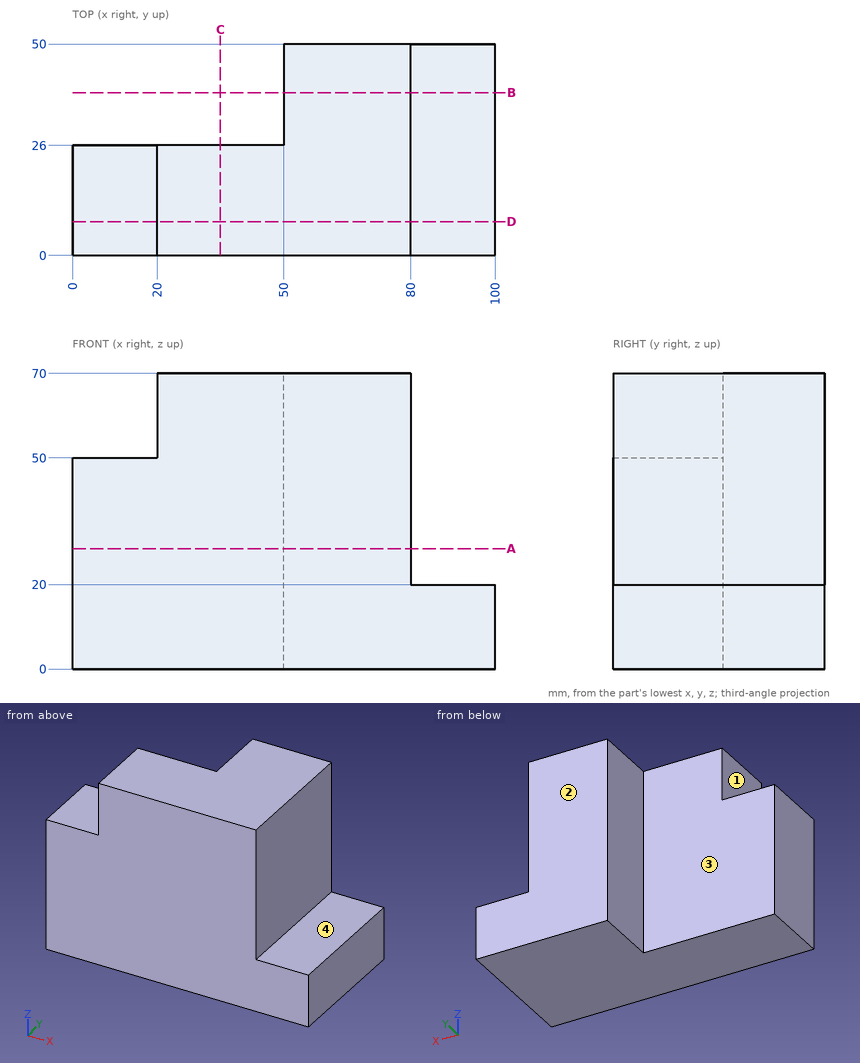
Answer from the drawing. Dimensions are ordinates in mm from the lowest x, y and z of the part. A direction names the side the tool comes from. Give positions to 0.01 mm unless a question says otherwise; leave off trailing zeros. Write each loop counter-clockwise with the first axis right and the second up, starting at its lowest first coordinate (ties: lowest second). Pieces come first, ordered by that corner, then holes. Notation, with made-up numbers: (-31, -22) -> (9, -22) arc R24 cw to (9, -10) -> close; hole circle Ø2 at (0, 8). An arc over 180 degrees is marked (long way). One line per question, with ' | ' between items. Start each with the question number.
1. Find the intervals of material crossed by probe 1 along X at (y, z) = (16, 29); probe 2 along Z at (x, y) = (93.5, 22); probe 3 along Y at (x, z) = (33.5, 32.5), in increasing order.
2. Section A-A (z = 28.5) is taken. Determine the outline of the cut face in (x, y), plus the area to 3 significant figures.
3. Section B-B (y = 38.5) is taken. Determine the outline of the cut face in (x, z).
4. Given pin 1 Ø22 at (x, y) = (92.5, 32) entering from +Z; pin 2 Ø12 at (x, z) = (21.5, 8) entering from +Y; pin 3 Ø19 at (y, z) = (36, 34.5) entering from -X, each flat-ended and moving along its own axis, determine where each tip first touches the part or whether it passes through.
5. Section C-C (x = 35) is taken. Determine the outline of the cut face in (y, z), plus the area to 3 significant figures.
6. For the marked faces 1, 2, 3 and 4, determine the directions among +Z, -Z, +X, -X, +Y, -Y from which every point of the face is accessible in a straight line to the end or side of a thin tool.
7. Section D-D (y = 8) is taken. Determine the outline of the cut face in (x, z), plus the area to 3 significant figures.
Response values:
1) probe 1: 0 to 80 | probe 2: 0 to 20 | probe 3: 0 to 26
2) outline: (0, 0) -> (80, 0) -> (80, 50) -> (50, 50) -> (50, 26) -> (0, 26) -> close | area: 2,800 mm2
3) outline: (50, 0) -> (100, 0) -> (100, 20) -> (80, 20) -> (80, 70) -> (50, 70) -> close
4) pin 1: z = 20 | pin 2: y = 26 | pin 3: x = 50
5) outline: (0, 0) -> (26, 0) -> (26, 70) -> (0, 70) -> close | area: 1,820 mm2
6) face 1: +Z, -X, +Y, -Y | face 2: +Z, -Z, +X, -X, +Y | face 3: +Z, -Z, -X, +Y | face 4: +Z, +X, +Y, -Y
7) outline: (0, 0) -> (100, 0) -> (100, 20) -> (80, 20) -> (80, 70) -> (20, 70) -> (20, 50) -> (0, 50) -> close | area: 5,600 mm2
